Work out the finished part from the listing and answer in its coordinate system (mm). Face numbers are marked on the shaded views. A direction names the side the tool comes from. Round coordinates to 2 decimals unless told otherwise and drop trailing zeros. Write each loop counter-clockwise with the first axis right and the second up, starting at its lowest first coordinate (ties: lowest second). Pieces come first, ordered by that corner, then holes. Notation, with made-up numbers: (33.5, -26.75) - (50.5, -26.75) arc R7 ccw to (50.5, -14.75) - close; hole circle Ø1 at (73, -7). An arc over 180 degrees is marked (long way). Answer as a JSON object with one key per item and string values.
```python
from build123d import *

# Parameters (mm, degrees)
BOSS_EXTRUDE1_DEPTH = 12.7
BOSS_EXTRUDE2_DEPTH = 6.35
SKETCH3_R           = 3.175
CUT_EXTRUDE1_DEPTH  = 12.7
CHAMFER1_SIZE       = 1.27


with BuildPart() as part:
    # Sketch1 → Boss-Extrude1 (new body)
    with BuildSketch(Plane(origin=(0, 0, 0), x_dir=(1, 0, 0), z_dir=(0, 1, 0))):
        with BuildLine():
            Line((279.4, 247.65), (279.4, 198.787506551))
            ThreePointArc((279.4, 198.787506551), (139.7, 118.11), (0, 198.787506551))
            Line((0, 198.787506551), (0, 247.65))
            ThreePointArc((0, 247.65), (139.7, 136.137470007), (279.4, 247.65))
        make_face()
    extrude(amount=BOSS_EXTRUDE1_DEPTH)

    # Sketch2 → Boss-Extrude2 (add)
    with BuildSketch(Plane.XZ):
        with BuildLine():
            Line((0, -198.787506551), (0, -159.420282964))
            ThreePointArc((0, -159.420282964), (139.7, -95.25), (279.4, -159.420282964))
            Line((279.4, -159.420282964), (279.4, -198.787506551))
            ThreePointArc((279.4, -198.787506551), (139.7, -118.11), (0, -198.787506551))
        make_face()
    extrude(amount=-BOSS_EXTRUDE2_DEPTH)

    # Sketch3 → Cut-Extrude1 (cut)
    with BuildSketch(Plane(origin=(0, 6.35, 0), x_dir=(1, 0, 0), z_dir=(0, 1, 0))):
        with Locations(Location((139.7, 106.68, 0), (0, 0, 270))):
            Circle(SKETCH3_R)
        with Locations(Location((25.4, 149.909813499, 0), (0, 0, 270))):
            Circle(SKETCH3_R)
        with Locations(Location((254, 149.909813499, 0), (0, 0, 270))):
            Circle(SKETCH3_R)
    extrude(amount=-CUT_EXTRUDE1_DEPTH, mode=Mode.SUBTRACT)

    # Chamfer1
    chamfer1_edges = [part.edges().sort_by_distance(p)[0] for p in [
        (139.7, 6.35, -109.855),
        (25.4, 6.35, -153.084813499),
        (254, 6.35, -153.084813499),
    ]]
    chamfer(chamfer1_edges, length=CHAMFER1_SIZE)


solid = part.part
```
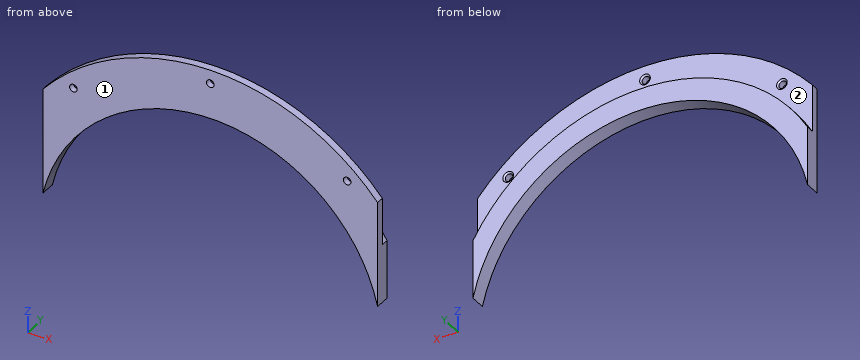
Item 1: A cutting plane is placed at C-C (y = 3). Write down the section's boundary in (x, z) (3 decimals), and give its area (3 significant figures).
Results found:
{"outline": "(0, -247.65) arc R143.263 cw to (279.4, -247.65) - (279.4, -159.42) arc R184.15 ccw to (0, -159.42) - close; hole circle Ø6.35 at (25.4, -149.91); hole circle Ø6.35 at (139.7, -106.68); hole circle Ø6.35 at (254, -149.91)", "area": "13,800 mm²"}
Item 2: Consider line 1 along X through (y, z) = (5, -218); line 2 along X through (y, z) = (8, -157.5); line 3 along Y through (x, z) = (235, -145.5). Determine where each line is inside the solid, lowest interval first.
Results found:
{"line 1": "0 to 10.26, 269.14 to 279.4", "line 2": "34.08 to 64.44, 214.96 to 245.32", "line 3": "0 to 6.35"}
Item 3: For the marked faces 1 and 2, determine the directions among +Z, -Z, +X, -X, +Y, -Y from which every point of the face is accessible in a straight line to the end or side of a thin tool.
Results found:
{"face 1": "+Z, -Z, +X, -X, -Y", "face 2": "+Z, +Y"}
Item 4: A cutting plane is placed at D-D (z = -106.68). Write down the section's boundary in (x, y) (3 decimals), and give its area (3 significant figures).
Results found:
{"outline": "(75.833, 0) - (136.525, 0) - (136.525, 5.08) - (135.255, 6.35) - (75.833, 6.35) - close; (142.875, 0) - (203.567, 0) - (203.567, 6.35) - (144.145, 6.35) - (142.875, 5.08) - close", "area": "769 mm²"}
Item 5: A cutting plane is placed at A-A (x = 139.7). Write down the section's boundary in (y, z) (3 decimals), and give its area (3 significant figures).
Results found:
{"outline": "(0, -136.137) - (12.7, -136.137) - (12.7, -118.11) - (6.35, -118.11) - (6.35, -111.125) - (5.08, -109.855) - (0, -109.855) - close; (0, -103.505) - (5.08, -103.505) - (6.35, -102.235) - (6.35, -95.25) - (0, -95.25) - close", "area": "332 mm²"}
Item 6: A cutting plane is placed at B-B (z = -193). Write down the section's boundary in (x, y).
Results found:
{"outline": "(0, 0) - (25.42, 0) - (25.42, 12.7) - (3.5, 12.7) - (3.5, 6.35) - (0, 6.35) - close; (253.98, 0) - (279.4, 0) - (279.4, 6.35) - (275.9, 6.35) - (275.9, 12.7) - (253.98, 12.7) - close"}
Item 7: Each of these flat-tipped pins is pushed along its axis until it touches: P1, Ø1, axis at y = 10.5, z = -151.5, coming from the -X side; P2, Ø2, axis at x = 213.5, y = 6.5, coming from the -Z side; P3, Ø10, axis at x = 25.4, z = -149.91, coming from the +Y side. Where does it stop, or does it pass through?
Results found:
{"P1": "x = 40.79", "P2": "z = -157.22", "P3": "y = 6.35"}
